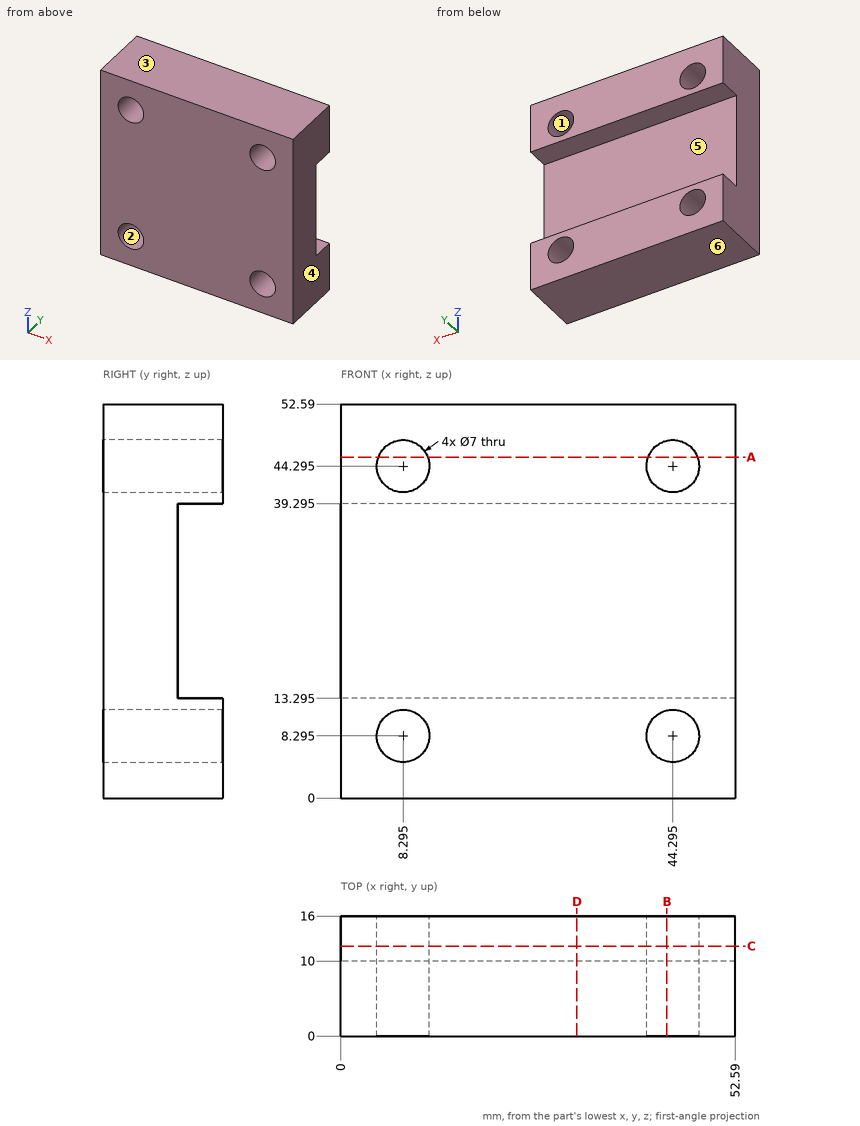
Study the drawing (mm; zero at the part's minimum x, y, z) and answer. A direction names the side the tool comes from. Give positions to 0.01 mm unless a question says otherwise; leave off trailing zeros. Write each loop counter-clockwise with the first axis right and the second up, starting at its lowest first coordinate (ties: lowest second). Pieces come first, ordered by that corner, then holes.
Item 1: Section B-B, the plane x = 43.5 is taken. Write down the section's boundary in (y, z) (3 decimals).
Item 2: Find the intervals of material crossed by line 1 along Z through (x, y) = (44, 2.25); line 2 along Z through (x, y) = (40, 12.25) (3 decimals); line 3 along X through (y, z) = (12.5, 11), in increasing order.
Item 3: Section C-C, the plane y = 12 is taken. Write down the section's boundary in (x, z) (3 decimals).
Item 4: Section A-A, the plane z = 45.5 is taken. Write down the section's boundary in (x, y), plus the area to 3 significant figures.
Item 5: Which of the six approach directions +Z, -Z, +X, -X, +Y, -Y give full straight-line access (tool end or side, diameter ignored) to the marked faces 5 and 6?
Item 6: Section D-D, the plane x = 31.5 is taken. Write down the section's boundary in (y, z) (3 decimals), plus the area to 3 significant figures.
Item 7: Flat-ended cylindrical pins translate along their axes: P1, Ø5.5, axis at x = 44.295, z = 44.295, coming from the +Y side; P2, Ø1, axis at x = 33.5, z = 31, coming from the +Y side. Find the tip coordinate at first contact, or state that the pin passes through.
Item 8: Determine the mould class of the marked faces 1, 2, 3 and 4 for opening direction X: released by +X, released by -X, zero draft, split by the parting line, or undercut.
Completed:
1. outline: (0, 0) - (16, 0) - (16, 4.886) - (0, 4.886) - close; (0, 11.704) - (16, 11.704) - (16, 13.295) - (10, 13.295) - (10, 39.295) - (16, 39.295) - (16, 40.886) - (0, 40.886) - close; (0, 47.704) - (16, 47.704) - (16, 52.59) - (0, 52.59) - close
2. line 1: z = 0 to 4.81, 11.78 to 40.81, 47.78 to 52.59
2. line 2: z = 0 to 13.295, 39.295 to 52.59
2. line 3: x = 0 to 6.07, 10.52 to 42.07, 46.52 to 52.59
3. outline: (0, 0) - (52.59, 0) - (52.59, 13.295) - (0, 13.295) - close; (0, 39.295) - (52.59, 39.295) - (52.59, 52.59) - (0, 52.59) - close; hole circle Ø7 at (8.295, 8.295); hole circle Ø7 at (8.295, 44.295); hole circle Ø7 at (44.295, 8.295); hole circle Ø7 at (44.295, 44.295)
4. outline: (0, 0) - (5.01, 0) - (5.01, 16) - (0, 16) - close; (11.58, 0) - (41.01, 0) - (41.01, 16) - (11.58, 16) - close; (47.58, 0) - (52.59, 0) - (52.59, 16) - (47.58, 16) - close
4. area: 631 mm2
5. face 5: +X, -X, +Y
5. face 6: -Z, +X, -X, +Y, -Y
6. outline: (0, 0) - (16, 0) - (16, 13.295) - (10, 13.295) - (10, 39.295) - (16, 39.295) - (16, 52.59) - (0, 52.59) - close
6. area: 685 mm2
7. P1: passes through
7. P2: stops at y = 10
8. face 1: undercut
8. face 2: undercut
8. face 3: zero draft
8. face 4: released by +X
